```python
from build123d import *

# Parameters (mm, degrees)
BOSS_EXTRUDE1_DEPTH = 12.7
CIRPATTERN1_COUNT   = 18
SKETCH3_W           = 2.032
SKETCH3_H           = 4.860083526
SKETCH5_R           = 1.905
BOSS_EXTRUDE3_DEPTH = 4.318
SKETCH6_R           = 5.855880208
CUT_EXTRUDE1_DEPTH  = 2.032
SKETCH7_R           = 4.2545
CUT_EXTRUDE2_DEPTH  = 95.903955419


with BuildPart() as part:
    # Sketch2 → Boss-Extrude1 (new body)
    with BuildSketch(Plane.XY):
        with BuildLine():
            Line((-4.887741292, -28.137706194), (-1.385764922, -28.755199114))
            ThreePointArc((-1.385764922, -28.755199114), (-1.335190156, -28.426609585), (-1.298996401, -28.09612676))
            Line((-1.298996401, -28.09612676), (-0.037512469, -28.206492303))
            ThreePointArc((-0.037512469, -28.206492303), (0.631557066, -28.119757595), (1.260329931, -27.875172976))
            ThreePointArc((1.260329931, -27.875172976), (1.27, -27.432), (1.260329931, -26.988827024))
            ThreePointArc((1.260329931, -26.988827024), (0.631557066, -26.744242405), (-0.037512469, -26.657507697))
            Line((-0.037512469, -26.657507697), (-1.298996401, -26.76787324))
            ThreePointArc((-1.298996401, -26.76787324), (-1.335190156, -26.437390415), (-1.385764922, -26.108800886))
            Line((-1.385764922, -26.108800886), (-4.887741292, -26.726293806))
            ThreePointArc((-4.887741292, -26.726293806), (-4.826, -27.432), (-4.887741292, -28.137706194))
        make_face()
    boss_extrude1 = extrude(amount=BOSS_EXTRUDE1_DEPTH)

    # CirPattern1: Boss-Extrude1 ×18 about axis
    cirpattern1_axis = Axis((-8.89, -27.432, 0), (0, 0, 1))
    for i in range(1, CIRPATTERN1_COUNT):
        add(boss_extrude1.rotate(cirpattern1_axis, i * 360 / CIRPATTERN1_COUNT))

    # Sketch3 → Cut-Revolve1 (revolve, cut)
    with BuildSketch(Plane(origin=(0, -27.432, 0), x_dir=(0, 0, -1), z_dir=(0, -1, 0))):
        with Locations((-11.684, -0.604078029)):
            Rectangle(SKETCH3_W, SKETCH3_H)
        with Locations((-1.016, -0.604078029)):
            Rectangle(SKETCH3_W, SKETCH3_H)
    revolve(axis=Axis((-8.89, -27.432, 12.7), (0, 0, -1)), mode=Mode.SUBTRACT)

    # Sketch5 → Boss-Extrude3 (add, symmetric)
    with BuildSketch(Plane.XY.offset(6.35)):
        with BuildLine():
            Line((-11.843249689, -32.488644073), (-75.646213327, -48.412823701))
            ThreePointArc((-75.646213327, -48.412823701), (-80.727352047, -45.361432), (-77.675960346, -40.280293281))
            Line((-77.675960346, -40.280293281), (-13.872996708, -24.356113653))
            ThreePointArc((-13.872996708, -24.356113653), (-14.571594361, -28.850033333), (-11.843249689, -32.488644073))
        make_face()
        with Locations((-76.661086837, -44.346558491)):
            Circle(SKETCH5_R, mode=Mode.SUBTRACT)
    extrude(amount=BOSS_EXTRUDE3_DEPTH, both=True)

    # Sketch6 → Cut-Extrude1 (cut)
    with BuildSketch(Plane(origin=(0, 0, 2.032), x_dir=(-1, 0, 0), z_dir=(0, 0, -1))):
        with Locations(Location((8.89, -27.432, 0), (0, 0, 180))):
            Circle(SKETCH6_R)
    extrude(amount=CUT_EXTRUDE1_DEPTH, mode=Mode.SUBTRACT)

    # Sketch7 → Cut-Extrude2 (cut, through all)
    with BuildSketch(Plane.XY.offset(12.7)):
        with Locations((-8.89, -27.432)):
            Circle(SKETCH7_R)
    extrude(amount=-CUT_EXTRUDE2_DEPTH, mode=Mode.SUBTRACT)


solid = part.part
```
Geometry check sheet. Reference: the model listing, model coordinates, mm. A direction names the side the tool comes from. Give positions to 0.01 mm unless a question says otherwise; leave off trailing zeros. Order: outer loops, then holes, each group sorted by start corner. A loop starts at its lowest first (then second) coordinate and runs counter-clockwise, first axis right, second up.
1. Section check B-B, the plane x = -58.5. Enter the section's corners in (y, z).
2. Release check for a two-part mould opening along Y. For faces 1 (the face through (-80.704, -45.451, 6.41)), 2 (the face through (-74.901, -45.076, 6.29)), 3 (the face through (-6.603, -23.845, 7.441)), 4 (the face through (-12, -24, 12.7)) record: pulls with the +Y half, pulls with the -Y half, needs draft (parallel to the pull), parting line crosses it, or undercut.
3. Gauge pin test, flat ends, axial feed: pin 1 Ø12 at (x, y) = (-40.5, -29.5) entering from -Z; pin 2 Ø2 at (x, z) = (-36, 3.5) entering from +Y; pin 3 Ø4 at (y, z) = (-21, 3) entering from -X; pin 4 Ø3 at (x, z) = (-27.5, 9.5) entering from -Y. Record the tip position at first contact, or that the pin passes through.
4. Access from +Z, -Z, +X, -X, +Y, -Y to the whole of each face (thin tool, end or side, straight path). Record for faces 5 (the face through (-6.188, -22.237, 11.67)), 6 (the face through (-6.56, -18.18, 6.29)), 7 (the face through (-45.839, -40.973, 6.41)), 8 (the face through (-40, -35, 2.032)).
5. Section check A-A, the plane y = -43.5. Enter the section's corners in (x, z), and give its area (3 significant figures).
6. Thickness scan on L1, parallel to X at y = -21.5, z = 8.5; L2, parallel to Y at x = -2, z = 7; L3, parallel to Z at x = -27.5, y = -32.5. Record the ranges inside material, lowest first.
7. Section check C-C, the plane z = 9.25. Give the number of separate pieces and of enclosed holes in the cut face, and give its area (3 significant figures).
Values follow:
1. outline: (-44.13, 2.03) - (-35.49, 2.03) - (-35.49, 10.67) - (-44.13, 10.67) - close
2. face 1: parting line crosses it
2. face 2: undercut
2. face 3: undercut
2. face 4: needs draft
3. pin 1: stops at z = 2.03
3. pin 2: stops at y = -29.63
3. pin 3: stops at x = -16.95
3. pin 4: stops at y = -36.77
4. face 5: +Z
4. face 6: +Z, -Z
4. face 7: +Z, -Z, -Y
4. face 8: -Z, +X, -X, +Y, -Y
5. outline: (-80.77, 2.03) - (-78.37, 2.03) - (-78.37, 10.67) - (-80.77, 10.67) - close; (-74.95, 2.03) - (-55.96, 2.03) - (-55.96, 10.67) - (-74.95, 10.67) - close
5. area: 185 mm2
6. L1: x = -16.83 to -14.82, -13.67 to -4.11, -2.96 to -0.95
6. L2: y = -34.1 to -32.26, -30.69 to -24.18, -22.61 to -20.77
6. L3: z = 2.03 to 10.67
7. separate pieces: 1
7. enclosed holes: 2
7. area: 720 mm2
